Build history of the part. All positions in model axes, mm. Round coordinates to 2 decimals unless told otherwise and drop trailing zeros. Order: outer loops, then holes, each group sorted by start corner. A loop starts at its lowest first (then second) coordinate and runs counter-clockwise, first axis right, second up. Notation, with made-up numbers: (85, 55) -> (98, 55) arc R11 cw to (98, 62) -> close; hole circle Ø6 at (36.5, 17). An arc over 180 degrees is marked (long way). Answer as a JSON object with one key per item and string values.
from build123d import *

# Parameters (mm, degrees)
SKETCH2_W           = 17
SKETCH2_H           = 7
BOSS_EXTRUDE1_DEPTH = 5
SKETCH3_W           = 20
SKETCH3_H           = 20
CUT_EXTRUDE1_DEPTH  = 5
BOSS_EXTRUDE2_DEPTH = 5


with BuildPart() as part:
    # Sketch2 → Boss-Extrude1 (new body)
    with BuildSketch(Plane(origin=(0, 0, 0), x_dir=(1, 0, 0), z_dir=(0, 1, 0))):
        Polygon((-44.718981883, -89.435737216), (45.281018117, -89.435737216), (45.281018117, 17.235484445), (75.281018117, 17.235484445), (75.281018117, 80.564262784), (-74.718981883, 80.564262784), (-74.718981883, 10.564262784), (-44.718981883, 10.564262784), align=None)
        with Locations((0.021018117, 72.514262784)):
            Rectangle(SKETCH2_W, SKETCH2_H, mode=Mode.SUBTRACT)
    extrude(amount=BOSS_EXTRUDE1_DEPTH)

    # Sketch3 → Cut-Extrude1 (cut)
    with BuildSketch(Plane(origin=(0, 5, 0), x_dir=(1, 0, 0), z_dir=(0, 1, 0))):
        Rectangle(SKETCH3_W, SKETCH3_H)
    extrude(amount=-CUT_EXTRUDE1_DEPTH, mode=Mode.SUBTRACT)

    # Sketch5 → Boss-Extrude2 (add)
    with BuildSketch(Plane(origin=(0, 5, 0), x_dir=(1, 0, 0), z_dir=(0, 1, 0))):
        Polygon((-39.650543722, -79.921839448), (40.212579957, -79.921839448), (40.212579957, -31.975199113), (45.281018117, -31.975199113), (45.281018117, -79.921839448), (45.281018117, -89.435737216), (-44.718981883, -89.435737216), (-44.718981883, -79.921839448), (-44.718981883, -31.975199113), (-39.650543722, -31.975199113), align=None)
    extrude(amount=BOSS_EXTRUDE2_DEPTH)


solid = part.part
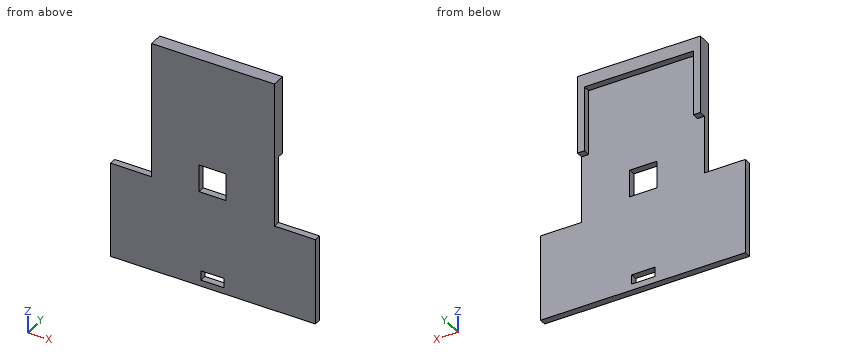
1) Flat gauge pins, fed straight in: pin 1 Ø4 at (x, y) = (-42.5, 8) entering from -Z; pin 2 Ø1.5 at (y, z) = (7, 54.5) entering from -X; pin 3 Ø4 at (x, z) = (-55, -57.5) entering from +Y. Where does each tip first touch, or does it go through?
Checked values:
{"pin 1": "stops at z = 31.98", "pin 2": "stops at x = -44.72", "pin 3": "stops at y = 5"}
2) Cut at D-D, the plane y = 8.5. Give the cut face in (x, z), plus the area to 3 significant figures.
Checked values:
{"outline": "(-44.72, 31.98) -> (-39.65, 31.98) -> (-39.65, 79.92) -> (40.21, 79.92) -> (40.21, 31.98) -> (45.28, 31.98) -> (45.28, 89.44) -> (-44.72, 89.44) -> close", "area": "1,340 mm²"}
3) Probe L1, parallel to Z at x = -8, y = 0.5; L2, parallel to X at y = 7, z = 76.5; L3, parallel to Z at x = -9, y = 3.75. List the from-to ranges inside material, lowest first. Write a range as from..to.
Checked values:
{"L1": "z = -80.56..-76.01, -69.01..-10, 10..89.44", "L2": "x = -44.72..-39.65, 40.21..45.28", "L3": "z = -80.56..-10, 10..89.44"}
4) Cut at A-A, the plane x = -6.5. Give the cut face in (y, z).
Checked values:
{"outline": "(0, -80.56) -> (5, -80.56) -> (5, -76.01) -> (0, -76.01) -> close; (0, -69.01) -> (5, -69.01) -> (5, -10) -> (0, -10) -> close; (0, 10) -> (5, 10) -> (5, 79.92) -> (10, 79.92) -> (10, 89.44) -> (0, 89.44) -> close"}
5) Cut at C-C, the plane z = 47.5. Give the cut face in (x, y), plus the area to 3 significant figures.
Checked values:
{"outline": "(-44.72, 0) -> (45.28, 0) -> (45.28, 10) -> (40.21, 10) -> (40.21, 5) -> (-39.65, 5) -> (-39.65, 10) -> (-44.72, 10) -> close", "area": "501 mm²"}
6) Cut at B-B, the plane z = 5.5. Give the cut face in (x, y), plus the area to 3 significant figures.
Checked values:
{"outline": "(-44.72, 0) -> (-10, 0) -> (-10, 5) -> (-44.72, 5) -> close; (10, 0) -> (45.28, 0) -> (45.28, 5) -> (10, 5) -> close", "area": "350 mm²"}
